Design review of the part built by this model. Coordinates are the model's own, in mm. Face numbers are marked on the shaded views. Give positions to 0.01 mm unless a question says otherwise; leave off trailing zeros. Loops run counter-clockwise (first coordinate to the right, second up) from the corner with the lowest first, then second, coordinate; pieces in that order, holes last. Notation, with made-up numbers: M -37.75,14.5 L -20.75,14.5 A23 cw -20.75,25.5 Z; hole C -7,-13 d5. An arc over 180 degrees is marked long. Use CSV: the item, a comma, the result in double quotes.
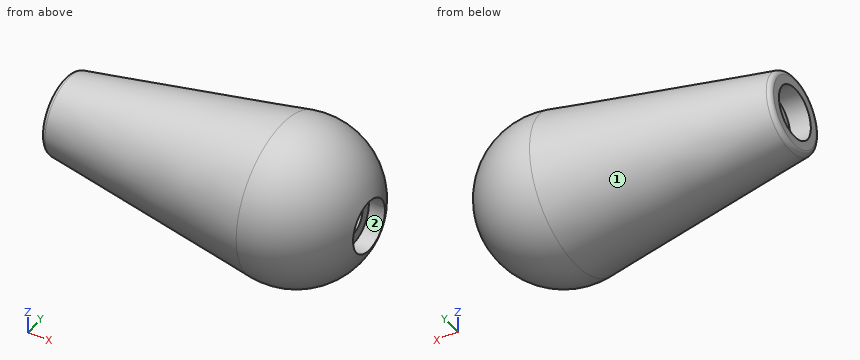
from build123d import *

# Parameters (mm, degrees)
FILLET1_R = 2


with BuildPart() as part:
    # Sketch1 → Revolve2 (revolve)
    with BuildSketch(Plane(origin=(0, 0, 0), x_dir=(1, 0, 0), z_dir=(0, 1, 0))):
        with BuildLine():
            Line((0, 0), (120, 0))
            ThreePointArc((120, 0), (109.337020363, 22.936426127), (84.928023767, 29.568142605))
            Line((84.928023767, 29.568142605), (0, 15))
            Line((0, 15), (0, 0))
        make_face()
    revolve(axis=Axis((0, 0, 0), (1, 0, 0)))

    # Sketch5 → Cut-Revolve1 (revolve, cut)
    with BuildSketch(Plane.XY):
        Polygon((0, 0), (0, 10), (8, 10), (8, 6), (112, 6), (112, 10), (120, 10), (120, 0), align=None)
    revolve(axis=Axis((120, 0, 0), (-1, 0, 0)), mode=Mode.SUBTRACT)

    # Fillet1
    fillet1_edges = [part.edges().sort_by_distance(p)[0] for p in [
        (0, 0, 15),
    ]]
    fillet(fillet1_edges, radius=FILLET1_R)


solid = part.part
(1) We need section C-C on x = 103. State the section outline as (y, z) points.
A:
outline,"C 0,0 d54.07; hole C 0,0 d12"
(2) Wall thickness on line 1 along Y through (x, z) = (91, 0); line 2 along Y through (x, z) = (5.5, 0); line 3 along Z through (x, y) = (6, 0): over which ranges is each line inside the solid? List them lowest first. Write a range as [from, to].
A:
line 1,"[-29.98, -6], [6, 29.98]"
line 2,"[-15.94, -10], [10, 15.94]"
line 3,"[-16.03, -10], [10, 16.03]"
(3) We need section D-D on x = 89.5. State the section outline as (y, z) points.
A:
outline,"C 0,0 d59.99; hole C 0,0 d12"
(4) Clearance check with flat-ended pins moving along their axes: P1, Ø1, axis at y = 2, z = 15.5, coming from the +X side; P2, Ø8, axis at y = 17.5, z = -2.5, coming from the +X side; P3, Ø2, axis at x = 85, z = 4, coming from the +Y side; P4, Ø3, axis at x = 28, y = -21.5, coming from the +Z side. State where each tip first meets the part, or that it passes through.
A:
P1,"x = 115.91"
P2,"x = 116.7"
P3,"y = 29.51"
P4,"through"
(5) We need section A-A on y = 0. State the section outline as (x, z) points.
A:
outline,"M 0,-13.31 A2 ccw 1.66,-15.29 L 84.93,-29.57 A30 ccw 118.28,-10 L 112,-10 L 112,-6 L 8,-6 L 8,-10 L 0,-10 Z; M 0,10 L 8,10 L 8,6 L 112,6 L 112,10 L 118.28,10 A30 ccw 84.93,29.57 L 1.66,15.29 A2 ccw 0,13.31 Z"
(6) The part is to be moulded in two halves that separate along Z. For the marked faces 1 and 2, say which applies: released by +Z, released by -Z, zero draft, split by the parting line, or undercut.
A:
face 1,"split by the parting line"
face 2,"undercut"
